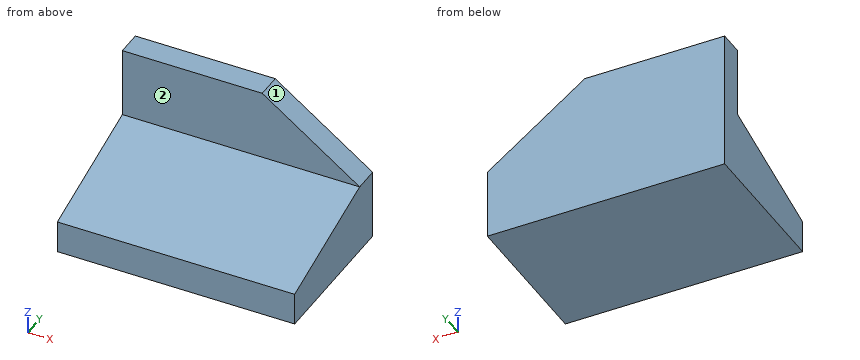
from build123d import *

# Parameters (mm, degrees)
F1_DEPTH = 95
F3_DEPTH = 25


with BuildPart() as f1:
    # F0 (on Right) → F1 (new body)
    with BuildSketch(Plane.YZ):
        Polygon((-60, 0), (0, 0), (0, 56), (-10, 56), (-10, 28), (-60, 13), align=None)
    extrude(amount=F1_DEPTH)

    # F2 (on face) → F3 (cut)
    with BuildSketch(Plane.XZ.offset(10)):
        Polygon((95, 56), (56, 56), (95, 28), align=None)
    extrude(amount=-F3_DEPTH, mode=Mode.SUBTRACT)


solid = f1.part
The listing builds one solid part. Answer for the finished solid, in the listing's coordinates (mm). Face numbers are marked on the shaded views. A direction names the side the tool comes from. Give positions to 0.01 mm unless a question says otherwise; leave off trailing zeros. Write each loop counter-clockwise with the first axis right and the second up, starting at its lowest first coordinate (ties: lowest second). Pieces come first, ordered by that corner, then holes.
Item 1: Section D-D, the plane y = -22.5 is taken. Write down the section's boundary in (x, z), plus the area to 3 significant figures.
Item 2: Which of the six approach directions +Z, -Z, +X, -X, +Y, -Y give full straight-line access (tool end or side, diameter ignored) to the marked faces 1 and 2?
Item 3: Find the intervals of material crossed by line 1 along Y through (x, z) = (24.5, 30); line 2 along X through (y, z) = (-9, 43); line 3 along Z through (x, y) = (54, -39.5), in increasing order.
Item 4: Section A-A, the plane y = -5.5 is taken. Write down the section's boundary in (x, z).
Item 5: Flat-ended cylindrical pins translate along their axes: P1, Ø2, axis at x = 71, y = -28.5, coming from the +Z side; P2, Ø6, axis at x = 61, y = -16, coming from the +Z side. Find the tip coordinate at first contact, or state that the pin passes through.
Item 6: Section B-B, the plane z = 35 is taken. Write down the section's boundary in (x, y), plus the area to 4 significant figures.
Item 7: Section C-C, the plane x = 21.5 is taken. Write down the section's boundary in (y, z), plus the area to 4 significant figures.
Completed:
1. outline: (0, 0) - (95, 0) - (95, 24.25) - (0, 24.25) - close
1. area: 2,300 mm2
2. face 1: +Z, +X, +Y, -Y
2. face 2: +Z, +X, -X, -Y
3. line 1: y = -10 to 0
3. line 2: x = 0 to 74.11
3. line 3: z = 0 to 19.15
4. outline: (0, 0) - (95, 0) - (95, 28) - (56, 56) - (0, 56) - close
5. P1: stops at z = 22.75
5. P2: stops at z = 27.1
6. outline: (0, -10) - (85.25, -10) - (85.25, 0) - (0, 0) - close
6. area: 852.5 mm2
7. outline: (-60, 0) - (0, 0) - (0, 56) - (-10, 56) - (-10, 28) - (-60, 13) - close
7. area: 1,585 mm2
